```python
from build123d import *

# Parameters (mm, degrees)
SKETCH1_R           = 3.5
BOSS_EXTRUDE1_DEPTH = 35
SKETCH2_R           = 12
BOSS_EXTRUDE2_DEPTH = 5
SKETCH3_R           = 0.2
CUT_EXTRUDE1_DEPTH  = 5
CIRPATTERN1_COUNT   = 20


with BuildPart() as part:
    # Sketch1 → Boss-Extrude1 (new body)
    with BuildSketch(Plane(origin=(0, 0, 0), x_dir=(1, 0, 0), z_dir=(0, 1, 0))):
        with Locations(Location((0, 0, 0), (0, 0, 270))):
            Circle(SKETCH1_R)
    extrude(amount=BOSS_EXTRUDE1_DEPTH)

    # Sketch2 → Boss-Extrude2 (add)
    with BuildSketch(Plane(origin=(0, 35, 0), x_dir=(1, 0, 0), z_dir=(0, 1, 0))):
        with Locations(Location((0, 0, 0), (0, 0, 270))):
            Circle(SKETCH2_R)
    extrude(amount=BOSS_EXTRUDE2_DEPTH)

    # Sketch3 → Cut-Extrude1 (cut)
    with BuildSketch(Plane(origin=(0, 40, 0), x_dir=(1, 0, 0), z_dir=(0, 1, 0))):
        with Locations(Location((0, 11, 0), (0, 0, 270))):
            Circle(SKETCH3_R)
    cut_extrude1 = extrude(amount=-CUT_EXTRUDE1_DEPTH, mode=Mode.SUBTRACT)

    # CirPattern1: Cut-Extrude1 ×20 about axis
    cirpattern1_axis = Axis((0, 0, 0), (0, 1, 0))
    for i in range(1, CIRPATTERN1_COUNT):
        add(cut_extrude1.rotate(cirpattern1_axis, i * 360 / CIRPATTERN1_COUNT), mode=Mode.SUBTRACT)


solid = part.part
```
Here's how the part is built. I have some questions about the finished solid (model axes, mm). A direction names the side the tool comes from. Coordinates: 2 decimals unless noted, no trailing zeros. Write each loop counter-clockwise with the first axis right and the second up, starting at its lowest first coordinate (ties: lowest second). Pieces come first, ordered by that corner, then holes. Notation, with made-up numbers: M 65,83 L 93,83 A19 ccw 93,106 Z; hole C 22,78.25 d6. An arc over 180 degrees is marked long. Answer as CSV lines item,"result". Start each with the question number.
Q1. Suppose I cut it at B-B, the plane y = 37. State how many separate pieces and enclosed holes the cut face has, then the cut area to 3 significant figures.
Q2. Suppose I cut it at C-C, the plane z = 1. List the corners of the cut face in (x, y) for me.
Q3. Will these pins go through, and if not, where does the flat tip stop? pin 1 Ø10 at (x, y) = (-5.5, 14) entering from -Z; pin 2 Ø8 at (x, z) = (-0.5, -8.5) entering from -Y; pin 3 Ø12 at (x, y) = (-8.5, 22.5) entering from -Z.
Q4. Suppose I cut it at D-D, the plane z = 5.5. List the corners of the cut face in (x, y) for me.
Q5. For faces 1 (the cylindrical face through (-3.417, 17.255, -0.759)), 2 (the flat face through (0, 40, 0)), which set-ups out of +Z, -Z, +X, -X, +Y, -Y let a thin tool reach every point of the face, with its end or its side?
Q6. I need wall thicknesses on probe 1 along Y at (x, z) = (6.25, -5.25); probe 2 along Z at (x, y) = (-2.5, 31); probe 3 along X at (y, z) = (37.9, -11). Which ranges of each line are inside material? Lowest first, please. Write a range as [from, to].
Q7. Suppose I cut it at A-A, the plane x = 1.5. List the corners of the cut face in (y, z) for me.
Entries:
1,separate pieces,"1"
1,enclosed holes,"20"
1,area,"450 mm²"
2,outline,"M -11.96,35 L -3.35,35 L -3.35,0 L 3.35,0 L 3.35,35 L 11.96,35 L 11.96,40 L -11.96,40 Z"
3,pin 1,"stops at z = -3.46"
3,pin 2,"stops at y = 35"
3,pin 3,"stops at z = -2.45"
4,outline,"M -10.67,35 L 10.67,35 L 10.67,40 L -10.67,40 Z"
5,face 1,"-Y"
5,face 2,"+Z, -Z, +X, -X, +Y"
6,probe 1,"y = [35, 40]"
6,probe 2,"z = [-2.45, 2.45]"
6,probe 3,"x = [-4.8, -0.2], [0.2, 4.8]"
7,outline,"M 0,-3.16 L 35,-3.16 L 35,-11.91 L 40,-11.91 L 40,11.91 L 35,11.91 L 35,3.16 L 0,3.16 Z"
